from build123d import *

# Parameters (mm, degrees)
EXTRUDE_1_DEPTH     = 15
EXTRUDE_2_DEPTH     = 3
SKETCH_3_R          = 4.4
CUT_EXTRUDE_1_DEPTH = 26.980762113533164
SKETCH_4_R          = 6.9
CUT_EXTRUDE_2_DEPTH = 9
CUT_EXTRUDE_3_DEPTH = 7
SKETCH_6_R          = 4.5
SKETCH_6_R_2        = 4.499999999999997
CUT_EXTRUDE_4_DEPTH = 2
FILLET_1_R          = 2


with BuildPart() as part:
    # Эскиз1 → Бобышка-Вытянуть1 (new body)
    with BuildSketch(Plane(origin=(0, 0, 0), x_dir=(1, 0, 0), z_dir=(0, 1, 0))):
        Polygon((14.999999999999998, 15.000000000000004), (-15.000000000000002, 15), (-14.999999999999998, -15), (15.000000000000002, -14.999999999999996), align=None)
    extrude(amount=EXTRUDE_1_DEPTH)

    # Эскиз2 → Бобышка-Вытянуть2 (add)
    with BuildSketch(Plane(origin=(0, 15, 0), x_dir=(1, 0, 0), z_dir=(0, 1, 0))):
        Polygon((-12.5, -2.499999999999997), (-15.000000000000002, -2.4999999999999973), (-15.000000000000002, 2.5000000000000027), (-12.5, 2.500000000000003), align=None)
        Polygon((15.000000000000002, -2.4999999999999973), (15.000000000000002, 2.5000000000000027), (12.5, 2.500000000000003), (12.5, -2.499999999999997), align=None)
    extrude(amount=EXTRUDE_2_DEPTH)

    # Эскиз3 → Вырез-Вытянуть1 (cut, through all)
    with BuildSketch(Plane(origin=(0, 15, 0), x_dir=(1, 0, 0), z_dir=(0, 1, 0))):
        with Locations(Location((0, 0, 0), (0, 0, 270))):
            Circle(SKETCH_3_R)
        with BuildLine():
            Line((-2.6, -15), (-2.6, -10))
            ThreePointArc((-2.6, -10), (1.6e-16, -7.4), (2.6, -10))
            Line((2.6, -10), (2.6, -15))
            Line((2.6, -15), (-2.6, -15))
        make_face()
        with BuildLine():
            Line((2.5999999999999974, 10), (2.6, 15))
            Line((2.6, 15), (-2.6, 15))
            Line((-2.6, 15), (-2.6000000000000023, 10))
            ThreePointArc((-2.6000000000000023, 10), (-2.93e-15, 7.4), (2.5999999999999974, 10))
        make_face()
    extrude(amount=-CUT_EXTRUDE_1_DEPTH, mode=Mode.SUBTRACT)

    # Эскиз4 → Вырез-Вытянуть2 (cut)
    with BuildSketch(Plane.XZ):
        with Locations(Location((0, 0, 0), (0, 0, 270))):
            Circle(SKETCH_4_R)
    extrude(amount=-CUT_EXTRUDE_2_DEPTH, mode=Mode.SUBTRACT)

    # Эскиз5 → Вырез-Вытянуть3 (cut)
    with BuildSketch(Plane(origin=(0, 15, 0), x_dir=(1, 0, 0), z_dir=(0, 1, 0))):
        with BuildLine():
            Line((-4.499999999999999, -15), (-4.5, -10))
            ThreePointArc((-4.5, -10), (2.8e-16, -5.5), (4.5, -10))
            Line((4.5, -10), (4.500000000000001, -15))
            Line((4.500000000000001, -15), (-4.499999999999999, -15))
        make_face()
        with BuildLine():
            Line((4.5, 10), (4.500000000000001, 15))
            Line((4.500000000000001, 15), (-4.499999999999999, 15))
            Line((-4.499999999999999, 15), (-4.5, 10))
            ThreePointArc((-4.5, 10), (-8.3e-16, 5.5), (4.5, 10))
        make_face()
    extrude(amount=-CUT_EXTRUDE_3_DEPTH, mode=Mode.SUBTRACT)

    # Эскиз6 → Вырез-Вытянуть4 (cut)
    with BuildSketch(Plane(origin=(0, 8, 0), x_dir=(1, 0, 0), z_dir=(0, 1, 0))):
        with Locations((0, -10)):
            Circle(SKETCH_6_R)
        with Locations((-2.45e-15, 10)):
            Circle(SKETCH_6_R_2)
    extrude(amount=-CUT_EXTRUDE_4_DEPTH, mode=Mode.SUBTRACT)

    # Скругление1
    fillet_1_edges = [part.edges().sort_by_distance(p)[0] for p in [
        (-15.000000000000002, 7.5, -15),
        (14.999999999999998, 7.5, -15.000000000000004),
        (15.000000000000002, 7.5, 14.999999999999996),
        (-14.999999999999998, 7.5, 15),
    ]]
    fillet(fillet_1_edges, radius=FILLET_1_R)


solid = part.part
Geometry: final body of the model. Coordinates: model frame, mm. A direction names the side the tool comes from. Give positions to 0.01 mm unless a question says otherwise; leave off trailing zeros. Write each loop counter-clockwise with the first axis right and the second up, starting at its lowest first coordinate (ties: lowest second). Pieces come first, ordered by that corner, then holes. Notation, with made-up numbers: M -20.75,-12 L -7.75,-12 A20 ccw -7.75,18 Z; hole C 41.25,68.5 d7. An arc over 180 degrees is marked long. Answer in a Markdown table with one row per item. Add a question column.
(1) Section C-C on x = 0. Return loops of the section in (y, z).
(2) Section B-B on z = 0. Return loops of the section in (x, y), and give its area (3 significant figures).
(3) Ray query, line 1 (X direction, y = 4.75, z = 0); line 2 (X direction, y = 11.55, z = 0); line 3 (Z direction, x = 0, y = 2). Return the intervals inside material, ascending.
(4) Reachability of faces 1 (the flat face through (5, 9, 0)), 2 (the flat face through (-2.6, 3, -13)), 3 (the flat face through (-4, 8, -14)) from +Z, -Z, +X, -X, +Y, -Y: full face, straight path, thin tool, end or side. Return the list, or none.
(5) Section D-D on y = 13.5. Return loops of the section in (x, z).
(6) Mould query, pull axis Z, two halves, no side actions, for faces 4 (the cylindrical face through (-0.159, 10.563, -5.503)), 5 (the cylindrical face through (4.363, 12.042, -0.573)), 6 (the flat face through (-14, 16, 2.5)), 7 (the flat face through (4.5, 12, -12)). Classes: +Z half, -Z half, draft (parallel to the pull), parting line (faces both ways), or undercut.
(7) First-contact query: pin 1 (1.5 mm diameter, centred on x = -3.5, z = 12, fed in from +Y); pin 2 (14 mm diameter, centred on x = 2, z = -2.5, fed in from -Y); pin 3 (0.8 mm diameter, centred on x = -14, y = 16.5, fed in from +Z); pin 4 (3.5 mm diameter, centred on x = 2, z = -9.5, fed in from +Y). Flat tips, straight axial feed; report the tip coordinate or a pass-through.
(8) Section A-A on y = 16.5. Return loops of the section in (x, z), and give its area (3 significant figures).
Result set:
| question | item | result |
|---|---|---|
| 1 | outline | M 0,-7.4 L 6,-7.4 L 6,-6.9 L 0,-6.9 Z; M 0,6.9 L 6,6.9 L 6,7.4 L 0,7.4 Z; M 9,-5.5 L 15,-5.5 L 15,-4.4 L 9,-4.4 Z; M 9,4.4 L 15,4.4 L 15,5.5 L 9,5.5 Z |
| 2 | outline | M -15,0 L -6.9,0 L -6.9,9 L -4.4,9 L -4.4,15 L -12.5,15 L -12.5,18 L -15,18 Z; M 4.4,9 L 6.9,9 L 6.9,0 L 15,0 L 15,18 L 12.5,18 L 12.5,15 L 4.4,15 Z |
| 2 | area | 288 mm^2 |
| 3 | line 1 | x = -15 to -6.9, 6.9 to 15 |
| 3 | line 2 | x = -15 to -4.4, 4.4 to 15 |
| 3 | line 3 | z = -7.4 to -6.9, 6.9 to 7.4 |
| 4 | face 1 | -Y |
| 4 | face 2 | -Z, +Y, -Y |
| 4 | face 3 | -Z, +Y |
| 5 | outline | M -15,-13 A2 ccw -13,-15 L -4.5,-15 L -4.5,-10 A4.5 cw 4.5,-10 L 4.5,-15 L 13,-15 A2 ccw 15,-13 L 15,13 A2 ccw 13,15 L 4.5,15 L 4.5,10 A4.5 cw -4.5,10 L -4.5,15 L -13,15 A2 ccw -15,13 Z; hole C 0,0 d8.8 |
| 6 | face 4 | undercut |
| 6 | face 5 | undercut |
| 6 | face 6 | +Z half |
| 6 | face 7 | draft |
| 7 | pin 1 | stops at y = 8 |
| 7 | pin 2 | stops at y = 0 |
| 7 | pin 3 | stops at z = 2.5 |
| 7 | pin 4 | stops at y = 6 |
| 8 | outline | M -15,-2.5 L -12.5,-2.5 L -12.5,2.5 L -15,2.5 Z; M 12.5,-2.5 L 15,-2.5 L 15,2.5 L 12.5,2.5 Z |
| 8 | area | 25.0 mm^2 |
